from build123d import *

# Parameters (mm, degrees)
BOSS_EXTRUDE1_DEPTH = 1
SKETCH2_W           = 14
SKETCH2_H           = 13
BOSS_EXTRUDE2_DEPTH = 7.5
SKETCH3_W           = 30
SKETCH3_H           = 20
SKETCH3_W_2         = 10
SKETCH3_H_2         = 11.389779098
BOSS_EXTRUDE3_DEPTH = 4
SKETCH5_W           = 17.510242059
SKETCH5_H           = 17.572802037
BOSS_EXTRUDE4_DEPTH = 4
SKETCH6_W           = 13
SKETCH6_H           = 14
BOSS_EXTRUDE5_DEPTH = 7.5
SKETCH7_W           = 16.2
SKETCH7_H           = 23.463684538
BOSS_EXTRUDE6_DEPTH = 7.5
SKETCH8_R           = 3
BOSS_EXTRUDE7_DEPTH = 9.5


with BuildPart() as part:
    # Sketch1 → Boss-Extrude1 (new body)
    with BuildSketch(Plane(origin=(0, 0, 0), x_dir=(1, 0, 0), z_dir=(0, 1, 0))):
        with BuildLine():
            Line((-29, 30), (29, 30))
            ThreePointArc((29, 30), (31.474873734, 28.974873734), (32.5, 26.5))
            Line((32.5, 26.5), (32.5, 3.5))
            ThreePointArc((32.5, 3.5), (31.474873734, 1.025126266), (29, 0))
            Line((29, 0), (-29, 0))
            ThreePointArc((-29, 0), (-31.474873734, 1.025126266), (-32.5, 3.5))
            Line((-32.5, 3.5), (-32.5, 26.5))
            ThreePointArc((-32.5, 26.5), (-31.474873734, 28.974873734), (-29, 30))
        make_face()
    extrude(amount=BOSS_EXTRUDE1_DEPTH)

    # Sketch2 → Boss-Extrude2 (add)
    with BuildSketch(Plane.XZ):
        with Locations((-18.811596296, -11.8)):
            Rectangle(SKETCH2_W, SKETCH2_H)
    extrude(amount=BOSS_EXTRUDE2_DEPTH)

    # Sketch3 → Boss-Extrude3 (add)
    with BuildSketch(Plane.XZ):
        with Locations((13.188403704, -11.795401308)):
            Rectangle(SKETCH3_W, SKETCH3_H)
        with Locations((-6.811596296, -11.795401308)):
            Rectangle(SKETCH3_W_2, SKETCH3_H_2)
    extrude(amount=BOSS_EXTRUDE3_DEPTH)

    # Sketch5 → Boss-Extrude4 (add)
    with BuildSketch(Plane.XZ.offset(4)):
        with Locations((8.67975542, -11.373546029)):
            Rectangle(SKETCH5_W, SKETCH5_H)
    extrude(amount=BOSS_EXTRUDE4_DEPTH)

    # Sketch6 → Boss-Extrude5 (add)
    with BuildSketch(Plane(origin=(0, 1, 0), x_dir=(1, 0, 0), z_dir=(0, 1, 0))):
        with Locations((0, 1.7)):
            Rectangle(SKETCH6_W, SKETCH6_H)
        with Locations((-17.6, 17.7)):
            Rectangle(SKETCH6_W, SKETCH6_H)
        with Locations((17.6, 17.7)):
            Rectangle(SKETCH6_W, SKETCH6_H)
    extrude(amount=BOSS_EXTRUDE5_DEPTH)

    # Sketch7 → Boss-Extrude6 (add)
    with BuildSketch(Plane(origin=(0, 1, 0), x_dir=(1, 0, 0), z_dir=(0, 1, 0))):
        with Locations((-17.444739374, -4.268157731)):
            Rectangle(SKETCH7_W, SKETCH7_H)
        with Locations((17.6, -4.268157731)):
            Rectangle(SKETCH7_W, SKETCH7_H)
    extrude(amount=BOSS_EXTRUDE6_DEPTH)

    # Sketch8 → Boss-Extrude7 (add)
    with BuildSketch(Plane.XY.offset(16)):
        with Locations(Location((-17.444739374, 4.75, 0), (0, 0, 180))):
            Circle(SKETCH8_R)
        with Locations(Location((17.6, 4.75, 0), (0, 0, 180))):
            Circle(SKETCH8_R)
    extrude(amount=BOSS_EXTRUDE7_DEPTH)


solid = part.part
Can you work these out from the model? Positions are in its coordinate system, mm. A direction names the side the tool comes from. Coordinates: 2 decimals unless noted, no trailing zeros. Order: outer loops, then holes, each group sorted by start corner. A loop starts at its lowest first (then second) coordinate and runs counter-clockwise, first axis right, second up. Notation, with made-up numbers: (-26.5, -13) -> (-2.5, -13) arc R27 cw to (-2.5, 16) -> close; hole circle Ø11 at (-34, 8). An arc over 180 degrees is marked (long way). Use one line per item in the form item = value.
Q1. I need wall thicknesses on L1, parallel to X at y = 2.5, z = -4; L2, parallel to Z at x = 22, y = 3; L3, parallel to X at y = 6.25, z = -19.5. Which ranges of each line are inside material? Lowest first, please.
From the geometry:
L1 = -25.54 to -9.34, -6.5 to 6.5, 9.5 to 25.7
L2 = -24.7 to -10.7, -7.46 to 16
L3 = -24.1 to -11.1, 11.1 to 24.1
Q2. Which directions (+Z, -Z, +X, -X, +Y, -Y) give clear straight access to the entire face, cutting with the end or side of a thin tool? Please do faces 1 (the face through (0, 5, -8.7)), 2 (the face through (-19, -7.5, -12)), 3 (the face through (-9.345, 5, 4)), 4 (the face through (0, 1, 3)).
From the geometry:
face_1 = -Z, +X, -X, +Y
face_2 = +Z, -Z, -X, -Y
face_3 = +Z, -Z, +Y
face_4 = +Z, +X, -X, -Y
Q3. Will these pins go through, and if not, where does the flat tip stop? P1, Ø3, axis at x = 15.5, y = -2.5, coming from the -Z side; P2, Ø4, axis at x = 2, z = 2.5, coming from the -Y side; P3, Ø4, axis at y = 4.5, z = -16.5, coming from the +X side; P4, Ø1.5, axis at x = -8, y = -0.5, coming from the -Z side.
From the geometry:
P1 = -21.8
P2 = 1
P3 = 24.1
P4 = -30
Q4. Imagine slicing it at D-D, the plane y = -1.5. List the corners of the cut face in (x, z) for me.
From the geometry:
outline = (-25.81, -18.3) -> (-11.81, -18.3) -> (-11.81, -17.49) -> (-1.81, -17.49) -> (-1.81, -21.8) -> (28.19, -21.8) -> (28.19, -1.8) -> (-1.81, -1.8) -> (-1.81, -6.1) -> (-11.81, -6.1) -> (-11.81, -5.3) -> (-25.81, -5.3) -> close
Q5. Imagine slicing it at A-A, the plane z = 13.5. List the corners of the cut face in (x, y) for me.
From the geometry:
outline = (-25.54, 1) -> (-9.34, 1) -> (-9.34, 8.5) -> (-25.54, 8.5) -> close; (9.5, 1) -> (25.7, 1) -> (25.7, 8.5) -> (9.5, 8.5) -> close
Q6. We'd pull the mould along X, two halves only. Please class faces 5 (the face through (-1.812, -2, -20)), 6 (the face through (13, -2, -21.795)), 7 (the face through (-31.5, 0.49, -28.95)): released by +X, released by -X, zero draft, split by the parting line, or undercut.
From the geometry:
face_5 = undercut
face_6 = zero draft
face_7 = released by -X
Q7. Imagine slicing it at B-B, the plane y = 4.75. List the corners of the cut face in (x, z) for me.
From the geometry:
outline = (-25.54, -7.46) -> (-9.34, -7.46) -> (-9.34, 16) -> (-14.44, 16) -> (-14.44, 25.5) -> (-20.44, 25.5) -> (-20.44, 16) -> (-25.54, 16) -> close; (-24.1, -24.7) -> (-11.1, -24.7) -> (-11.1, -10.7) -> (-24.1, -10.7) -> close; (-6.5, -8.7) -> (6.5, -8.7) -> (6.5, 5.3) -> (-6.5, 5.3) -> close; (9.5, -7.46) -> (25.7, -7.46) -> (25.7, 16) -> (20.6, 16) -> (20.6, 25.5) -> (14.6, 25.5) -> (14.6, 16) -> (9.5, 16) -> close; (11.1, -24.7) -> (24.1, -24.7) -> (24.1, -10.7) -> (11.1, -10.7) -> close
Q8. Imagine slicing it at C-C, the plane x = 5. List the corners of the cut face in (y, z) for me, then the cut area to 3 significant figures.
From the geometry:
outline = (-8, -20.16) -> (-4, -20.16) -> (-4, -21.8) -> (0, -21.8) -> (0, -30) -> (1, -30) -> (1, -8.7) -> (8.5, -8.7) -> (8.5, 5.3) -> (1, 5.3) -> (1, 0) -> (0, 0) -> (0, -1.8) -> (-4, -1.8) -> (-4, -2.59) -> (-8, -2.59) -> close
area = 285 mm²
